from build123d import *

# Parameters (mm, degrees)
ESQUISSE1_W                  = 65
ESQUISSE1_H                  = 200
ESQUISSE1_R                  = 1
BOSS_EXTRU_1_DEPTH           = 10
ESQUISSE2_W                  = 65
ESQUISSE2_H                  = 15
BOSS_EXTRU_2_DEPTH           = 30
ESQUISSE3_W                  = 41
ESQUISSE3_H                  = 20
ENL_V_MAT_EXTRU_1_DEPTH      = 215.067746286
ENL_V_MAT_EXTRU_2_DEPTH      = 178
ENL_V_MAT_EXTRU_2_DEPTH_BACK = 8
ESQUISSE4_W                  = 55
ESQUISSE4_H                  = 20
ESQUISSE5_R                  = 1
ENL_V_MAT_EXTRU_3_DEPTH      = 215.067746286
ESQUISSE6_W                  = 10
ESQUISSE6_H                  = 120
ENL_V_MAT_EXTRU_4_DEPTH      = 10


with BuildPart() as part:
    # Esquisse1 → Boss.-Extru.1 (new body)
    with BuildSketch(Plane.XY):
        with Locations((-32.5, -100)):
            Rectangle(ESQUISSE1_W, ESQUISSE1_H)
        with Locations((-55, -25)):
            Circle(ESQUISSE1_R, mode=Mode.SUBTRACT)
        with Locations((-45, -40)):
            Circle(ESQUISSE1_R, mode=Mode.SUBTRACT)
        with Locations((-20, -40)):
            Circle(ESQUISSE1_R, mode=Mode.SUBTRACT)
        with Locations((-10, -25)):
            Circle(ESQUISSE1_R, mode=Mode.SUBTRACT)
        with Locations((-45, -160)):
            Circle(ESQUISSE1_R, mode=Mode.SUBTRACT)
        with Locations((-20, -160)):
            Circle(ESQUISSE1_R, mode=Mode.SUBTRACT)
        with Locations((-10, -175)):
            Circle(ESQUISSE1_R, mode=Mode.SUBTRACT)
        with Locations((-55, -175)):
            Circle(ESQUISSE1_R, mode=Mode.SUBTRACT)
    extrude(amount=BOSS_EXTRU_1_DEPTH)

    # Esquisse2 → Boss.-Extru.2 (add)
    with BuildSketch(Plane.XY.offset(10)):
        with Locations((-32.5, -7.5)):
            Rectangle(ESQUISSE2_W, ESQUISSE2_H)
        with Locations((-32.5, -192.5)):
            Rectangle(ESQUISSE2_W, ESQUISSE2_H)
    extrude(amount=BOSS_EXTRU_2_DEPTH)

    # Esquisse3 → Enlèv. mat.-Extru.1 (cut, through all)
    with BuildSketch(Plane.XZ.offset(200)):
        with Locations((-32.5, 25)):
            Rectangle(ESQUISSE3_W, ESQUISSE3_H)
    extrude(amount=-ENL_V_MAT_EXTRU_1_DEPTH, mode=Mode.SUBTRACT)

    # Esquisse4 → Enlèv. mat.-Extru.2 (cut, two sides: drawn at the far end of the back side and taken through both)
    with BuildSketch(Plane.XZ.offset(15).offset(-ENL_V_MAT_EXTRU_2_DEPTH_BACK)):
        with Locations((-32.5, 25)):
            Rectangle(ESQUISSE4_W, ESQUISSE4_H)
    extrude(amount=ENL_V_MAT_EXTRU_2_DEPTH + ENL_V_MAT_EXTRU_2_DEPTH_BACK, mode=Mode.SUBTRACT)

    # Esquisse5 → Enlèv. mat.-Extru.3 (cut, through all)
    with BuildSketch(Plane.XY.offset(40)):
        with Locations((-55, -12)):
            Circle(ESQUISSE5_R)
        with Locations((-10, -12)):
            Circle(ESQUISSE5_R)
        with Locations((-10, -188)):
            Circle(ESQUISSE5_R)
        with Locations((-55, -188)):
            Circle(ESQUISSE5_R)
    extrude(amount=-ENL_V_MAT_EXTRU_3_DEPTH, mode=Mode.SUBTRACT)

    # Esquisse6 → Enlèv. mat.-Extru.4 (cut)
    with BuildSketch(Plane.XY.offset(10)):
        with Locations((-60, -100)):
            Rectangle(ESQUISSE6_W, ESQUISSE6_H)
        with Locations((-5, -100)):
            Rectangle(ESQUISSE6_W, ESQUISSE6_H)
    extrude(amount=-ENL_V_MAT_EXTRU_4_DEPTH, mode=Mode.SUBTRACT)


solid = part.part
Part model, mm, in its own coordinate system. A direction names the side the tool comes from. Round coordinates to 2 decimals unless told otherwise and drop trailing zeros. Write each loop counter-clockwise with the first axis right and the second up, starting at its lowest first coordinate (ties: lowest second). Pieces come first, ordered by that corner, then holes. Notation, with made-up numbers: M -25,4.25 L 14,4.25 A13 cw 14,25.25 Z; hole C 44,5 d7. An arc over 180 degrees is marked long. Return JSON: item names as keys, results as strings. Group by question number.
(1) Saw through at D-D on y = -178. Write the cut outline in (x, z), then the cut area to 3 significant figures.
(2) Drill centre lines: probe 1 along Y at (x, z) = (-20, 6.25); probe 2 along X at (y, z) = (-188, 6); probe 3 along Y at (x, z) = (-11, 28). Where is each one in solid material? Low to high.
(3) Which spindle directions (+Z, -Z, +X, -X, +Y, -Y) get a long thin tool onto all of the face, cutting with end or side? Do faces 1 (the face through (-60, -189, 25)), 2 (the face through (-5, -160, 5)), 3 (the face through (-33, -185, 14.8)), 4 (the face through (-53, -197, 25)). Say none if no direction does.
(4) Saw through at C-C on y = -152.5. Write the cut outline in (x, z).
(5) Saw through at A-A on z = 32. Write the cut outline in (x, y), then the cut area to 3 significant figures.
(6) Saw through at B-B on z = 5. Count the separate pieces of the cut face and the enclosed holes in it, then the cut area to 3 significant figures.
(7) Pin check, flat tips, straight feed: pin 1 Ø11 at (y, z) = (-78.5, 6.5) entering from -X; pin 2 Ø19.5 at (x, y) = (-48.5, -59) entering from +Z; pin 3 Ø5 at (y, z) = (-107.5, 4) entering from +X. Stop position of each tip, or through.
(8) Two-plate mould, pull along X, no slides. Class faces 5 (the face through (-55, -101, 5)), 6 (the face through (-33, -200, 11)), 7 (the face through (-33, -193, 35)): +X half, -X half, draft (parallel to the pull), parting line (faces both ways), or undercut.
Returned:
{
 "1": {"outline": "M -65,0 L 0,0 L 0,10 L -65,10 Z", "area": "650 mm²"},
 "2": {"probe 1": "-200 to -161, -159 to -41, -39 to 0", "probe 2": "-65 to -56, -54 to -11, -9 to 0", "probe 3": "-200 to -193, -7 to 0"},
 "3": {"face 1": "none", "face 2": "+Z, -Z, +X", "face 3": "+Z, +X, -X", "face 4": "+Y, -Y"},
 "4": {"outline": "M -55,0 L -10,0 L -10,10 L -55,10 Z"},
 "5": {"outline": "M -65,-200 L -53,-200 L -53,-193 L -60,-193 L -60,-185 L -65,-185 Z; M -65,-15 L -60,-15 L -60,-7 L -53,-7 L -53,0 L -65,0 Z; M -12,-200 L 0,-200 L 0,-185 L -5,-185 L -5,-193 L -12,-193 Z; M -12,-7 L -5,-7 L -5,-15 L 0,-15 L 0,0 L -12,0 Z", "area": "496 mm²"},
 "6": {"separate pieces": "1", "enclosed holes": "12", "area": "10,600 mm²"},
 "7": {"pin 1": "x = -55", "pin 2": "z = 10", "pin 3": "x = -10"},
 "8": {"face 5": "-X half", "face 6": "draft", "face 7": "undercut"}
}
